Solid Edge part; units mm, degrees
sketch "Sketch1" plane through (0, 0, 0) normal (0, -1, 0) x (1, 0, 0)
  line L0 (-69.1361, 133.121) -> (-44.1361, 133.121)
  line L1 (-44.1361, 133.121) -> (-44.1361, -26.879)
  line L2 (-44.1361, -26.879) -> (-49.1361, -26.879)
  line L3 (-49.1361, 128.121) -> (-49.1361, -26.879)
  line L4 (-64.1361, 128.121) -> (-49.1361, 128.121)
  line L5 (-64.1361, -26.879) -> (-64.1361, 128.121)
  line L6 (-64.1361, -26.879) -> (-69.1361, -26.879)
  line L7 (-69.1361, -26.879) -> (-69.1361, 133.121)
extrude "Protrusion1" add sketch "Sketch1" against normal blind 80
fillet "Round_1" radius 5 2 edges at (-69.1361, 40, 133.121) (-44.1361, 40, 133.121)
fillet "Round_2" radius 5 2 edges at (-64.1361, 40, 128.121) (-49.1361, 40, 128.121)
sketch "Sketch2" plane through (-44.1361, 40, 18.121) normal (1, 0, 0) x (0, 1, 0)
  circle A0 centre (-25, -30) radius 5
  circle A1 centre (25, -30) radius 5
  circle A2 centre (0, 46) radius 7.5
  dimension "D1" = 25
extrude "Cutout1" cut sketch "Sketch2" against normal through all
Input: part model. Units: mm. Frame: model coordinates. A direction names the side the tool comes from. Give positions to 0.01 mm unless a question says otherwise; leave off trailing zeros. Loops run counter-clockwise (first coordinate to the right, second up) from the corner with the lowest first, then second, coordinate; pieces in that order, holes last. Notation, with made-up numbers: M 18.25,79 L 24.25,79 A6 ccw 24.25,84 Z; hole C 57.25,-11 d9. An arc over 180 degrees is marked long. Answer as CSV lines item,"result". Start each with the question number.
1. Section C-C on y = 31. Return loops of the section in (x, z), plus the area to 4 significant figures.
2. Pull-direction query (X, two-part tool) for faces 3 (the face through (-45.64, 40.56, 131.695)), 4 (the face through (-67, 39, -26.879)), 5 (the face through (-62.71, 40.56, 126.62)); classes: released by +X, released by -X, zero draft, split by the parting line, or undercut.
3. Reachability of faces 1 (the face through (-46.601, 39.024, 71.557)), 2 (the face through (-64.136, 39, 47)) from +Z, -Z, +X, -X, +Y, -Y: full face, straight path, thin tool, end or side. Return the list, or none.
4. Section B-B on y = 40. Return loops of the section in (x, z).
5. Section D-D on y = 15. Return loops of the section in (x, z), plus the area to 4 significant figures.
6. Section A-A on z = 90. Return loops of the section in (x, y).
7. Pin query (flat end, axial travel): P1, Ø10, axis at x = -56.5, z = 9, coming from the -Y side; P2, Ø4, axis at x = -56.5, y = 29, coming from the -Z side. Return the tip coordinate at first contact, or that it passes through.
8. Line query: L1, parallel to X at y = 38, z = 50; L2, parallel to Z at x = -45.25, y = 35.5; L3, parallel to Z at x = -67.9, y = 15. Output: solid intervals per line, ascending.
Computed values:
1,outline,"M -69.14,-26.88 L -64.14,-26.88 L -64.14,123.12 A5 cw -59.14,128.12 L -54.14,128.12 A5 cw -49.14,123.12 L -49.14,-26.88 L -44.14,-26.88 L -44.14,128.12 A5 ccw -49.14,133.12 L -64.14,133.12 A5 ccw -69.14,128.12 Z"
1,area,"1,675 mm²"
2,face 3,"released by +X"
2,face 4,"zero draft"
2,face 5,"undercut"
3,face 1,"+X, -X"
3,face 2,"-Z, +Y, -Y"
4,outline,"M -69.14,-26.88 L -64.14,-26.88 L -64.14,56.62 L -69.14,56.62 Z; M -69.14,71.62 L -64.14,71.62 L -64.14,123.12 A5 cw -59.14,128.12 L -54.14,128.12 A5 cw -49.14,123.12 L -49.14,71.62 L -44.14,71.62 L -44.14,128.12 A5 ccw -49.14,133.12 L -64.14,133.12 A5 ccw -69.14,128.12 Z; M -49.14,-26.88 L -44.14,-26.88 L -44.14,56.62 L -49.14,56.62 Z"
5,outline,"M -69.14,-26.88 L -64.14,-26.88 L -64.14,-16.88 L -69.14,-16.88 Z; M -69.14,-6.88 L -64.14,-6.88 L -64.14,123.12 A5 cw -59.14,128.12 L -54.14,128.12 A5 cw -49.14,123.12 L -49.14,-6.88 L -44.14,-6.88 L -44.14,128.12 A5 ccw -49.14,133.12 L -64.14,133.12 A5 ccw -69.14,128.12 Z; M -49.14,-26.88 L -44.14,-26.88 L -44.14,-16.88 L -49.14,-16.88 Z"
5,area,"1,575 mm²"
6,outline,"M -69.14,0 L -64.14,0 L -64.14,80 L -69.14,80 Z; M -49.14,0 L -44.14,0 L -44.14,80 L -49.14,80 Z"
7,P1,"passes through"
7,P2,"stops at z = 128.12"
8,L1,"x = -69.14 to -64.14, -49.14 to -44.14"
8,L2,"z = -26.88 to 58.12, 70.12 to 131.27"
8,L3,"z = -26.88 to -16.88, -6.88 to 131.41"
